Geometry: final body of the model. Coordinates: model frame, mm. A direction names the side the tool comes from. Round coordinates to 2 decimals unless told otherwise and drop trailing zeros. Write each loop counter-clockwise with the first axis right and the second up, starting at its lowest first coordinate (ties: lowest second). Pieces come first, ordered by that corner, then holes. Notation, with made-up numbers: (68, 16.25) - (89, 16.25) arc R18 cw to (89, 40.25) - close; hole circle Ø2 at (77.25, 75). An arc over 180 degrees is marked (long way). Write each question's results on one line, items separated by ' | '.
from build123d import *

# Parameters (mm, degrees)
SKETCH1_R           = 30
BOSS_EXTRUDE1_DEPTH = 5
SKETCH2_R           = 2.65
CUT_EXTRUDE1_DEPTH  = 2.6


with BuildPart() as part:
    # Sketch1 → Boss-Extrude1 (new body, symmetric)
    with BuildSketch(Plane(origin=(0, 0, 0), x_dir=(1, 0, 0), z_dir=(0, 1, 0))):
        Circle(SKETCH1_R)
    extrude(amount=BOSS_EXTRUDE1_DEPTH, both=True)

    # Sketch2 → Cut-Extrude1 (cut, symmetric)
    with BuildSketch(Plane(origin=(0, 0, 0), x_dir=(1, 0, 0), z_dir=(0, 1, 0))):
        with Locations((-12.5, 12.5)):
            Circle(SKETCH2_R)
        with Locations((12.5, 12.5)):
            Circle(SKETCH2_R)
        with Locations((12.5, -12.5)):
            Circle(SKETCH2_R)
        with Locations((-12.5, -12.5)):
            Circle(SKETCH2_R)
    extrude(amount=CUT_EXTRUDE1_DEPTH, both=True, mode=Mode.SUBTRACT)


solid = part.part
Q1. Section query B-B, the plane z = -12.5. Return loops of the section in (x, y), plus the area to 3 significant figures.
Answer block:
outline: (-27.27, -5) - (27.27, -5) - (27.27, 5) - (-27.27, 5) - close; hole (-15.15, -2.6) - (-9.85, -2.6) - (-9.85, 2.6) - (-15.15, 2.6) - close; hole (9.85, -2.6) - (15.15, -2.6) - (15.15, 2.6) - (9.85, 2.6) - close | area: 490 mm2
Q2. Access query for faces 1 (the flat face through (12, -2.6, -13)), 2 (the cylindrical face through (-29.97, 0.07, -1.32)). Directions: +Z, -Z, +X, -X, +Y, -Y. A direction counts if a zero-diameter tool reaches every point of the face in a straight line with its end or side. Return the directions, or none.
Answer block:
face 1: none | face 2: +Y, -Y
Q3. Ray query, line 1 along X through (y, z) = (0.05, 12.5); line 2 along Z through (x, y) = (-13.5, 0). Return the intervals inside material, ascending.
Answer block:
line 1: -27.27 to -15.15, -9.85 to 9.85, 15.15 to 27.27 | line 2: -26.79 to -14.95, -10.05 to 10.05, 14.95 to 26.79
Q4. Section query C-C, the plane y = -0.5. Return loops of the section in (x, z), plus the area to 3 significant figures.
Answer block:
outline: circle Ø60 at (0, 0); hole circle Ø5.3 at (-12.5, -12.5); hole circle Ø5.3 at (-12.5, 12.5); hole circle Ø5.3 at (12.5, -12.5); hole circle Ø5.3 at (12.5, 12.5) | area: 2,740 mm2
Q5. Section query D-D, the plane y = 3.5. Return loops of the section in (x, z), plus the area to 3 significant figures.
Answer block:
outline: circle Ø60 at (0, 0) | area: 2,830 mm2
Q6. Pin query (flat end, axial travel): pin 1 (2 mm diameter, centred on y = 2.5, z = 6.5, fed in from -X). Return the tip coordinate at first contact, or that it passes through.
Answer block:
pin 1: x = -29.49
Q7. Mould query, pull axis Y, two halves, no side actions, for faces 3 (the flat face through (-13, 2.6, -13)), 4 (the flat face through (0, -5, 0)), 5 (the flat face through (-13, -2.6, -13)), 6 (the flat face through (0, 5, 0)). Classes: pulls with the +Y half, pulls with the -Y half, needs draft (parallel to the pull), parting line crosses it, or undercut.
Answer block:
face 3: undercut | face 4: pulls with the -Y half | face 5: undercut | face 6: pulls with the +Y half
Q8. Section query A-A, the plane x = 12.5. Return loops of the section in (y, z).
Answer block:
outline: (-5, -27.27) - (5, -27.27) - (5, 27.27) - (-5, 27.27) - close; hole (-2.6, -15.15) - (2.6, -15.15) - (2.6, -9.85) - (-2.6, -9.85) - close; hole (-2.6, 9.85) - (2.6, 9.85) - (2.6, 15.15) - (-2.6, 15.15) - close
